```python
from build123d import *

# Parameters (mm, degrees)
SKETCH1_W           = 136
SKETCH1_H           = 90
BOSS_EXTRUDE1_DEPTH = 24
SKETCH4_R           = 0.930895073
SKETCH4_W           = 13.5
SKETCH4_H           = 5
SKETCH4_W_2         = 9.671745291
SKETCH4_H_2         = 12.631347156
SKETCH4_R_2         = 3.3980858
CUT_EXTRUDE1_DEPTH  = 10
SKETCH3_W           = 50
SKETCH3_H           = 9
CUT_EXTRUDE2_DEPTH  = 10
SKETCH2_R           = 3.5
SKETCH2_W           = 80
SKETCH2_H           = 7
CUT_EXTRUDE3_DEPTH  = 10
FILLET1_R           = 8
CHAMFER1_SIZE       = 3
CUT_EXTRUDE4_DEPTH  = 5
CUT_EXTRUDE5_START  = 73.8
CUT_EXTRUDE5_DEPTH  = 2
LPATTERN1_COUNT     = 8
LPATTERN1_PITCH     = 5.8
SKETCH7_W           = 73
SKETCH7_H           = 50
CUT_EXTRUDE6_DEPTH  = 1


# Read off the part's stored shape, not the designer's step: Cut-Extrude5
with BuildPart() as part:
    # Sketch1 → Boss-Extrude1 (new body)
    with BuildSketch(Plane(origin=(0, 0, 0), x_dir=(1, 0, 0), z_dir=(0, 1, 0))):
        with Locations((68, 45)):
            Rectangle(SKETCH1_W, SKETCH1_H)
    extrude(amount=BOSS_EXTRUDE1_DEPTH)

    # Sketch4 → Cut-Extrude1 (cut)
    # profile 1 of 4: a face of its own
    with BuildSketch(Plane(origin=(136, 0, 0), x_dir=(0, 0, -1), z_dir=(1, 0, 0))):
        with Locations((78.971843902, 12)):
            Circle(SKETCH4_R)
    # profile 2 of 4: a face of its own
    with BuildSketch(Plane(origin=(136, 0, 0), x_dir=(0, 0, -1), z_dir=(1, 0, 0))):
        Polygon((37.51037714, 10), (37.51037714, 16.5), (39.01037714, 18), (45.01037714, 18), (46.51037714, 16.5), (46.51037714, 10), align=None)
    # profile 3 of 4: a face of its own
    with BuildSketch(Plane(origin=(136, 0, 0), x_dir=(0, 0, -1), z_dir=(1, 0, 0))):
        with Locations((23.357700282, 12)):
            Rectangle(SKETCH4_W, SKETCH4_H)
    # profile 4 of 4: a face of its own
    with BuildSketch(Plane(origin=(136, 0, 0), x_dir=(0, 0, -1), z_dir=(1, 0, 0))):
        with Locations((70.687922275, 12.465761788)):
            Rectangle(SKETCH4_W_2, SKETCH4_H_2)
        with Locations((70.707468534, 13.819380659)):
            Circle(SKETCH4_R_2, mode=Mode.SUBTRACT)
    extrude(amount=-CUT_EXTRUDE1_DEPTH, mode=Mode.SUBTRACT)

    # Sketch3 → Cut-Extrude2 (cut)
    with BuildSketch(Plane(origin=(0, 0, -90), x_dir=(-1, 0, 0), z_dir=(0, 0, -1))):
        with Locations((-38, 12)):
            Rectangle(SKETCH3_W, SKETCH3_H)
        with Locations((-98, 12)):
            Rectangle(SKETCH3_W, SKETCH3_H)
    extrude(amount=-CUT_EXTRUDE2_DEPTH, mode=Mode.SUBTRACT)

    # Sketch2 → Cut-Extrude3 (cut)
    with BuildSketch(Plane.XY):
        with Locations((33, 15.5)):
            Circle(SKETCH2_R)
        with Locations((22, 15.5)):
            Circle(SKETCH2_R)
        with Locations((81, 12)):
            Rectangle(SKETCH2_W, SKETCH2_H)
    extrude(amount=-CUT_EXTRUDE3_DEPTH, mode=Mode.SUBTRACT)

    # Fillet1
    fillet1_edges = [part.edges().sort_by_distance(p)[0] for p in [
        (0, 12, -90),
        (136, 12, -90),
        (136, 12, 0),
        (0, 12, 0),
    ]]
    fillet(fillet1_edges, radius=FILLET1_R)

    # Chamfer1
    chamfer1_edges = [part.edges().sort_by_distance(p)[0] for p in [
        (0, 0, -45),
        (0, 24, -45),
        (68, 0, -90),
        (136, 0, -45),
        (68, 0, 0),
        (133.656854249, 0, -87.656854249),
        (133.656854249, 0, -2.343145751),
        (2.343145751, 0, -2.343145751),
        (2.343145751, 0, -87.656854249),
        (68, 24, -90),
        (68, 24, 0),
        (136, 24, -45),
        (133.656854249, 24, -87.656854249),
        (133.656854249, 24, -2.343145751),
        (2.343145751, 24, -2.343145751),
        (2.343145751, 24, -87.656854249),
    ]]
    chamfer(chamfer1_edges, length=CHAMFER1_SIZE)

    # Sketch5 → Cut-Extrude4 (cut)
    with BuildSketch(Plane.XZ):
        with BuildLine():
            Line((32.8, -43), (27.264101615, -43))
            ThreePointArc((27.264101615, -43), (19.8, -45), (27.264101615, -47))
            Line((27.264101615, -47), (32.8, -47))
            ThreePointArc((32.8, -47), (34.8, -45), (32.8, -43))
        make_face()
        with BuildLine():
            Line((112.8, -24.9), (107.264101615, -24.9))
            ThreePointArc((107.264101615, -24.9), (99.8, -22.9), (107.264101615, -20.9))
            Line((107.264101615, -20.9), (112.8, -20.9))
            ThreePointArc((112.8, -20.9), (114.8, -22.9), (112.8, -24.9))
        make_face()
        with BuildLine():
            Line((112.8, -65.1), (107.264101615, -65.1))
            ThreePointArc((107.264101615, -65.1), (99.8, -67.1), (107.264101615, -69.1))
            Line((107.264101615, -69.1), (112.8, -69.1))
            ThreePointArc((112.8, -69.1), (114.8, -67.1), (112.8, -65.1))
        make_face()
    extrude(amount=-CUT_EXTRUDE4_DEPTH, mode=Mode.SUBTRACT)

    # Cut-Extrude5 outline → Cut-Extrude5 (cut)
    with BuildSketch(Plane.YZ.offset(CUT_EXTRUDE5_START)):
        Polygon((21, 0), (19.585786438, 0), (24, -4.414213562), (24, -3), align=None)
    cut_extrude5 = extrude(amount=CUT_EXTRUDE5_DEPTH, mode=Mode.SUBTRACT)

    # LPattern1: Cut-Extrude5 ×8, 1 skipped
    with Locations(*[(i * LPATTERN1_PITCH, 0, 0) for i in range(1, LPATTERN1_COUNT) if i not in (4,)]):
        add(cut_extrude5, mode=Mode.SUBTRACT)

    # Sketch7 → Cut-Extrude6 (cut)
    with BuildSketch(Plane(origin=(0, 24, 0), x_dir=(1, 0, 0), z_dir=(0, 1, 0))):
        with Locations((67.5, 45)):
            Rectangle(SKETCH7_W, SKETCH7_H)
    extrude(amount=-CUT_EXTRUDE6_DEPTH, mode=Mode.SUBTRACT)


solid = part.part
```
Geometry check sheet. Reference: the model listing, model coordinates, mm. A direction names the side the tool comes from. Coordinates: 2 decimals unless noted, no trailing zeros. Loops run counter-clockwise (first coordinate to the right, second up) from the corner with the lowest first, then second, coordinate; pieces in that order, holes last.
Item 1: Thickness scan on line 1 (Y direction, x = 81, z = -84.5); line 2 (X direction, y = 8.5, z = -83.5); line 3 (Z direction, x = 23.8, y = 3.5). Record the ranges inside material, lowest first.
Item 2: Release check for a two-part mould opening along Y. For faces 1 (the face through (38, 16.5, -85)), 2 (the face through (69, 1, -2)), 3 (the face through (67, 23, -45)) record: released by +Y, released by -Y, zero draft, split by the parting line, or undercut.
Item 3: Sectioned sample at B-B, the plane x = 23.8. Record the boundary of the cut face in (y, z), then the cut area to 3 significant figures.
Item 4: Access from +Z, -Z, +X, -X, +Y, -Y to the whole of each face (thin tool, end or side, straight path). Record for faces 4 (the face through (131, 9.5, -23)), 5 (the face through (110, 2, -20.9)), 6 (the face through (3.702, 22.854, -3.607)), 7 (the face through (85.4, 22, -2)), 8 (the face through (36.34, 16.55, -4.93)).
Item 5: Sectioned sample at C-C, the plane z = -84. Count the separate pieces of the cut face and the enclosed holes in it, then the cut area to 3 significant figures.
Item 6: Go/stop test with flat-tipped pins: pin 1 Ø5 at (x, z) = (103.8, -67.1) entering from -Y; pin 2 Ø1.5 at (x, y) = (23, 13) entering from -Z; pin 3 Ø1.1 at (x, y) = (59, 23.5) entering from +Z. Record where each tip stops, or that it passes through.
Item 7: Sectioned sample at A-A, the plane z = -60.5. Record the boundary of the cut face in (x, y).
Check result:
1. line 1: y = 0 to 7.5, 16.5 to 24
1. line 2: x = 0.14 to 13, 63 to 73, 123 to 135.86
1. line 3: z = -90 to -49, -41 to 0
2. face 1: undercut
2. face 2: released by -Y
2. face 3: released by +Y
3. outline: (0, -87) - (3, -90) - (7.5, -90) - (7.5, -80) - (16.5, -80) - (16.5, -90) - (21, -90) - (24, -87) - (24, -3) - (21, 0) - (18.5, 0) - (18.5, -10) - (12.5, -10) - (12.5, 0) - (3, 0) - (0, -3) - (0, -41) - (5, -41) - (5, -49) - (0, -49) - close
3. area: 1,950 mm2
4. face 4: +X
4. face 5: -Y
4. face 6: +Z, -X, +Y
4. face 7: +Z, +Y
4. face 8: +Z
5. separate pieces: 1
5. enclosed holes: 2
5. area: 2,330 mm2
6. pin 1: stops at y = 5
6. pin 2: stops at z = -80
6. pin 3: stops at z = -1.95
7. outline: (0, 3) - (3, 0) - (133, 0) - (136, 3) - (136, 21) - (133, 24) - (104, 24) - (104, 23) - (31, 23) - (31, 24) - (3, 24) - (0, 21) - close
